Input: part model. Units: mm. Frame: model coordinates. Give positions to 0.01 mm unless a question says otherwise; leave off trailing zeros. Order: outer loops, then holes, each group sorted by start corner. A loop starts at its lowest first (then second) coordinate and runs counter-clockwise, first axis right, second up. Notation, with made-up numbers: M 57.5,-32 L 92.5,-32 A10 ccw 92.5,-18 Z; hole C -34,-9 d5. An arc over 180 degrees is marked long. Use a Markdown table: item, result.
from build123d import *

# Parameters (mm, degrees)
EXTRUDE_1_DEPTH   = 2
HOLE_WIZARD_M81_D = 9
CHAMFER_1_SIZE    = 2


with BuildPart() as part:
    # Эскиз1 → Бобышка-Вытянуть1 (new body)
    with BuildSketch(Plane(origin=(0, 0, 0), x_dir=(1, 0, 0), z_dir=(0, 0, -1))):
        Polygon((-40, 120), (40, 120), (40, 80), (20, 80), (20, 0), (-20, 0), (-20, 80), (-40, 80), align=None)
    extrude(amount=EXTRUDE_1_DEPTH)

    # Отверстие с зазором M81 (through all)
    with Locations(Plane(origin=(0, 0, -2), x_dir=(1, 0, 0), z_dir=(0, 0, -1))):
        with Locations((20, 100), (0, 60), (0, 20), (-20, 100)):
            Hole(HOLE_WIZARD_M81_D / 2)

    # Фаска1
    chamfer_1_edges = [part.edges().sort_by_distance(p)[0] for p in [
        (-40, -80, -1),
        (-40, -120, -1),
        (40, -120, -1),
        (40, -80, -1),
        (20, 0, -1),
        (-20, 0, -1),
    ]]
    chamfer(chamfer_1_edges, length=CHAMFER_1_SIZE)


solid = part.part
1) Cut plane C-C on z = -1.6. Return loops of the section in (x, y).
Response values:
| item | result |
|---|---|
| outline | M -40,-118 L -38,-120 L 38,-120 L 40,-118 L 40,-82 L 38,-80 L 20,-80 L 20,-2 L 18,0 L -18,0 L -20,-2 L -20,-80 L -38,-80 L -40,-82 Z; hole C -20,-100 d9; hole C 0,-60 d9; hole C 0,-20 d9; hole C 20,-100 d9 |
2) Cut plane B-B on y = -20. Return loops of the section in (x, z), and give its area (3 significant figures).
Response values:
| item | result |
|---|---|
| outline | M -20,-2 L -4.5,-2 L -4.5,0 L -20,0 Z; M 4.5,-2 L 20,-2 L 20,0 L 4.5,0 Z |
| area | 62.0 mm² |
3) Cut plane A-A on x = 0. Return loops of the section in (y, z), and give its area (3 significant figures).
Response values:
| item | result |
|---|---|
| outline | M -120,-2 L -64.5,-2 L -64.5,0 L -120,0 Z; M -55.5,-2 L -24.5,-2 L -24.5,0 L -55.5,0 Z; M -15.5,-2 L 0,-2 L 0,0 L -15.5,0 Z |
| area | 204 mm² |
4) Material intervals for line 1 (X direction, y = -100, z = -0.85); line 2 (Y direction, x = 0, z = -1.25); line 3 (X direction, y = -60, z = -1), sorted ascending. Write a range as from..to.
Response values:
| item | result |
|---|---|
| line 1 | x = -40..-24.5, -15.5..15.5, 24.5..40 |
| line 2 | y = -120..-64.5, -55.5..-24.5, -15.5..0 |
| line 3 | x = -20..-4.5, 4.5..20 |
5) Cut plane D-D on x = 22.5. Return loops of the section in (y, z), and give its area (3 significant figures).
Response values:
| item | result |
|---|---|
| outline | M -120,-2 L -103.74,-2 L -103.74,0 L -120,0 Z; M -96.26,-2 L -80,-2 L -80,0 L -96.26,0 Z |
| area | 65.0 mm² |
6) First-contact query: pin 1 Ø1 at (y, z) = (-52.5, -1.5) entering from +X; pin 2 Ø0.6 at (x, z) = (28.5, -1) entering from +Y. Flat tips, straight axial feed; report the tip coordinate or a pass-through.
Response values:
| item | result |
|---|---|
| pin 1 | stops at x = 20 |
| pin 2 | stops at y = -80 |
